Model file for the job. Use its own axes, mm. Face numbers are marked on the shaded views. A direction names the side the tool comes from. Coordinates: 2 decimals unless noted, no trailing zeros. Order: outer loops, then holes, each group sorted by start corner. A loop starts at its lowest first (then second) coordinate and runs counter-clockwise, first axis right, second up.
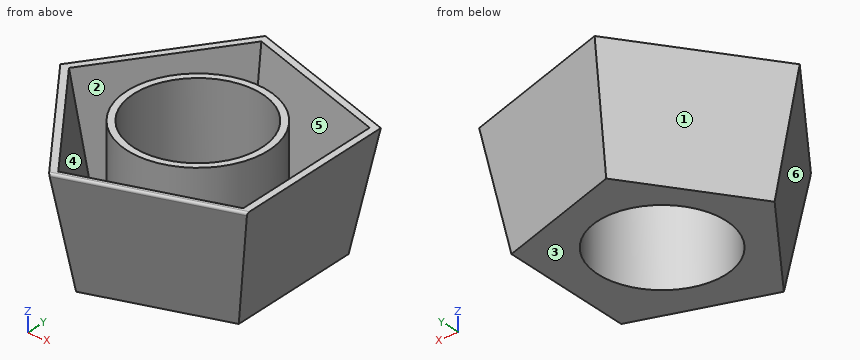
Autodesk Fusion 360 part; units mm, degrees
sketch "스케치1" plane through (0, 0, 0) normal (0, 0, 1) x (1, 0, 0)
  line L0 (-15, 6) -> (-22, -7)
  line L1 (-22, -7) -> (-9, -9)
  line L2 (-9, -9) -> (-3, 0)
  line L3 (-3, 0) -> (-12, 7)
  line L4 (3, 5) -> (3, -9.4098)
  line L5 (3, -9.4098) -> (20.2982, -14.6076)
  line L6 (20.2982, -14.6076) -> (26.171, 4.9371)
  line L7 (26.171, 4.9371) -> (7.7071, 8.424)
  line L8 (42.6307, 4.9371) -> (42, -15)
  line L9 (42, -15) -> (67.9355, -17.567)
  line L10 (67.9355, -17.567) -> (65.6256, 5.8006)
  line L11 (65.6256, 5.8006) -> (42.6307, 4.9371)
  line L12 (78.9292, 2.5635) -> (78.4348, -13.0662)
  line L13 (78.4348, -13.0662) -> (106, -18)
  arc A0 (106, -18) -> (78.9292, 2.5635) centre (112.5801, 18.7627) ccw
  line L14 (-78.1892, -7.301) -> (-40, -7.301)
  line L15 (-40, -7.301) -> (-40, 37.2455)
  arc A1 (-40, 37.2455) -> (-75, 40) centre (-57.6084, 37.2455) ccw
  line L16 (-75, 40) -> (-75, -7.301)
  line L17 (-75, -25) -> (-35, -25)
  line L18 (-35, -25) -> (-35, -65)
  line L19 (-35, -65) -> (-75, -65)
  line L20 (-75, -65) -> (-75, -25)
  line L21 (20, -31.5) -> (70, -31.5)
  line L22 (70, -31.5) -> (70, -81.5)
  line L23 (70, -81.5) -> (20, -81.5)
  line L24 (20, -81.5) -> (20, -31.5)
  curve L25
  curve L26
  curve L27
  curve L28
  curve L29 construction
  curve L30 construction
  line L31 (221.7769, -77.0241) -> (180.313, -77.0241)
  line L32 (180.313, -77.0241) -> (180.313, -31.5347)
  line L33 (180.313, -31.5347) -> (221.7769, -31.5347)
  line L34 (221.7769, -31.5347) -> (221.7769, -77.0241)
  line L35 (221.7769, -77.0241) -> (180.313, -31.5347) construction
  line L36 (180.313, -77.0241) -> (221.7769, -31.5347) construction
  circle A2 centre (-30, -160) radius 25.461
  circle A3 centre (27.6815, -165.0053) radius 31.7614
  circle A4 centre (125.6318, -141.5124) radius 31.894
  circle A5 centre (125.6318, -141.5124) radius 31.894
  circle A6 centre (157.3931, -144.4186) radius 36.4671
  circle A7 centre (190.6677, -144.4186) radius 5.5401
  circle A8 centre (152.4397, -176.5897) radius 12.8987
  circle A9 centre (125.6318, -192.8529) radius 43.2366
  circle A10 centre (125.6318, -173.4064) radius 27.8792
  line L37 (-174.3672, -75.4378) -> (-188.8141, -19.5395)
  line L38 (-188.8141, -19.5395) -> (-244.4468, -4.1017)
  line L39 (-244.4468, -4.1017) -> (-285.6328, -44.5622)
  line L40 (-285.6328, -44.5622) -> (-271.1859, -100.4605)
  line L41 (-271.1859, -100.4605) -> (-215.5532, -115.8983)
  line L42 (-215.5532, -115.8983) -> (-174.3672, -75.4378)
  line L43 (-160.849, -213.9216) -> (-162.0762, -155.1559)
  line L44 (-162.0762, -155.1559) -> (-218.345, -138.1635)
  line L45 (-218.345, -138.1635) -> (-251.8938, -186.4273)
  line L46 (-251.8938, -186.4273) -> (-216.3593, -233.2484)
  line L47 (-216.3593, -233.2484) -> (-160.849, -213.9216)
  point P0 (201.045, -54.2794)
  point P1 (-230, -60)
  point P2 (-201.9047, -185.3833)
  dimension "d1" = 40
  dimension "d2" = 40
  dimension "d3" = 50
  dimension "d4" = 50
  dimension "d5" = 50
  dimension "d6" = 60
  dimension "d7" = 60
  dimension "d8" = 60
  dimension "d9" = 50
  dimension "d10" = 50
extrude "돌출1" add sketch "스케치1" along normal blind 50 draft 10 contours L43 L44 L45 L46 L47
sketch "스케치2" plane through (0, 0, 50) normal (0, 0, 1) x (-1, 0, 0)
  circle A0 centre (203.6154, 184.7621) radius 27.8241
extrude "돌출2" cut sketch "스케치2" against normal blind 50
shell "쉘1" thickness 3 removed faces 1 at (-160.3626, -184.4905, 50)
fillet "필렛1" radius 1 2 edges at (-185.7053, -231.9111, 50) (-186.7069, -229.0342, 50)
Q1. Mould opens along Y. For the marked faces 3, 4, 5 and 6 say: pulls with the +Y half, pulls with the -Y half, needs draft (parallel to the pull), parting line crosses it, or undercut.
Established:
face 3: needs draft
face 4: undercut
face 5: undercut
face 6: pulls with the -Y half
Q2. Which spindle directions (+Z, -Z, +X, -X, +Y, -Y) get a long thin tool onto all of the face, cutting with end or side? Do the marked faces 1 and 2. Say none if no direction does.
Established:
face 1: -Z, -X, +Y
face 2: +Z
Q3. Cut at C-C, the plane x = -228.5. List the corners of the cut face in (y, z).
Established:
outline: (-231.83, 50) - (-217.25, 0) - (-197.21, 0) - (-197.21, 50) - (-202.95, 50) - (-202.95, 3) - (-213.09, 3) - (-226.8, 50) - close; (-172.31, 0) - (-152.77, 0) - (-137.33, 50) - (-142.66, 50) - (-157.18, 3) - (-166.57, 3) - (-166.57, 50) - (-172.31, 50) - close
Q4. Drop flat-ended pins along their axis: P1, Ø4, axis at x = -163, z = 30.5, coming from the +Y side; P2, Ø6, axis at x = -240.5, z = 17.5, coming from the +Y side; P3, Ø1.5, axis at x = -220, z = 11.5, coming from the -Y side. Give the stop position or say it passes through.
Established:
P1: stops at y = -148.55
P2: stops at y = -160.22
P3: stops at y = -232.82
Q5. Cut at A-A, the plane z = 32.5. List the corners of the cut face in (x, y), plus the area to 3 significant figures.
Established:
outline: (-258.98, -186.58) - (-218.41, -240.03) - (-155.03, -217.96) - (-156.43, -150.87) - (-220.67, -131.47) - close; circle Ø61.65 at (-203.62, -184.76); hole (-255.21, -186.5) - (-217.32, -236.42) - (-158.12, -215.82) - (-159.43, -153.15) - (-219.44, -135.03) - close; hole circle Ø55.65 at (-203.62, -184.76)
area: 1,540 mm2
Q6. Cut at D-D, the plane z = 23.5. List the corners of the cut face in (x, y) (1 decimal).
Established:
outline: (-257, -186.5) - (-217.8, -238.2) - (-156.6, -216.8) - (-158, -152.1) - (-220, -133.3) - close; circle Ø61.6 at (-203.6, -184.8); hole (-253.2, -186.5) - (-216.8, -234.5) - (-159.7, -214.7) - (-161, -154.3) - (-218.8, -136.9) - close; hole circle Ø55.6 at (-203.6, -184.8)
Q7. Cut at B-B, the plane y = -182.5. List the corners of the cut face in (x, z), plus the area to 3 significant figures.
Established:
outline: (-259.9, 50) - (-249.16, 0) - (-231.35, 0) - (-231.35, 50) - (-234.36, 50) - (-234.36, 3) - (-246.1, 3) - (-256.19, 50) - close; (-175.88, 0) - (-161.51, 0) - (-152.69, 50) - (-155.73, 50) - (-164.02, 3) - (-172.87, 3) - (-172.87, 50) - (-175.88, 50) - close
area: 699 mm2
Q8. Probe line 1 (X direction, y = -181.5, z = 41); line 2 (X direction, y = -213, z = 10); line 3 (Y direction, x = -186.5, z = 34.5). List the from-to ranges inside material, lowest first.
Established:
line 1: x = -257.27 to -253.56, -234.27 to -231.25, -175.98 to -172.96, -157.34 to -154.3
line 2: x = -233.94 to -230.12, -215.97 to -191.26, -162.15 to -159.1
line 3: y = -229.29 to -226.07, -210.4 to -206.7, -162.82 to -159.13, -144.61 to -141.43
